Design review of the part built by this model. Coordinates are the model's own, in mm. Face numbers are marked on the shaded views. A direction names the side the tool comes from. Round coordinates to 2 decimals unless told otherwise and drop trailing zeros. Write each loop counter-clockwise with the first axis right and the second up, starting at its lowest first coordinate (ties: lowest second). Pieces come first, ordered by that corner, then holes. Notation, with made-up numbers: (15, -40) -> (34, -40) arc R29 cw to (34, -13) -> close; hole circle Ø10 at (-13, 26.5). An arc over 180 degrees is marked (long way). One line per question, with ' | ' between items. Start each with the question number.
1) Consider section C-C (x = 0). Give the boundary of the cut face in (y, z), then the cut area to 3 significant figures.
2) For the marked faces 1 and 2, list the 3-axis set-ups (+Z, -Z, +X, -X, +Y, -Y) from which the entire face can be reached by the end or side of a thin tool; tool diameter is ignored.
3) For probe 1 along X at (y, z) = (18, 0.25); probe 2 along Y at (x, z) = (9.75, -0.75); probe 3 along Z at (x, y) = (-8, 18), list the stretches that pass through material, from the lowest coordinate up.
4) Consider section B-B (x = -8). Give the boundary of the cut face in (y, z).
5) Consider section D-D (y = 26). Give the boundary of the cut face in (x, z), then the cut area to 3 significant figures.
6) Consider section A-A (z = 0). Give the boundary of the cut face in (x, y), then the cut area to 3 significant figures.
7) Insertion check: pin 1 Ø12 at (x, z) = (-4, 7.5) entering from -Y; pin 2 Ø3 at (x, y) = (11.5, 25.5) entering from -Z; pin 3 Ø2 at (x, z) = (12, -0.5) entering from -Y; pin 4 Ø9 at (x, z) = (-2.5, -1.5) entering from -Y. Each pin has a flat end and moves straight along its axis. Give the tip position at first contact, or say it passes through.
```python
from build123d import *

# Parameters (mm, degrees)
F0_R     = 15
F0_R_2   = 1.25
F0_R_3   = 5.5
F1_DEPTH = 45
F2_DEPTH = 2
F3_R     = 1.6
F4_DEPTH = 9


with BuildPart() as f1:
    # F0 (on Front) → F1 (new body)
    with BuildSketch(Plane.XZ):
        Circle(F0_R)
        with Locations((-8, 0)):
            Circle(F0_R_2, mode=Mode.SUBTRACT)
        Circle(F0_R_3, mode=Mode.SUBTRACT)
        with Locations((8, 0)):
            Circle(F0_R_2, mode=Mode.SUBTRACT)
        Circle(F0_R_3)
    extrude(amount=-F1_DEPTH)

    # F0 (on Front) → F2 (join)
    with BuildSketch(Plane.XZ):
        Circle(F0_R_3)
    extrude(amount=F2_DEPTH)

    # F3 (on face) → F4 (join)
    with BuildSketch(Plane.XZ.offset(2)):
        Circle(F3_R)
    extrude(amount=F4_DEPTH)


solid = f1.part
```
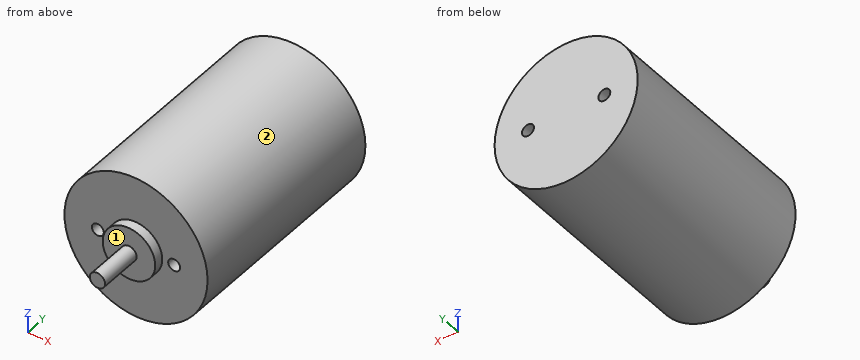
From the geometry:
1) outline: (-11, -1.6) -> (-2, -1.6) -> (-2, -5.5) -> (0, -5.5) -> (0, -15) -> (45, -15) -> (45, 15) -> (0, 15) -> (0, 5.5) -> (-2, 5.5) -> (-2, 1.6) -> (-11, 1.6) -> close | area: 1,400 mm2
2) face 1: -Y | face 2: +Y, -Y
3) probe 1: x = -15 to -9.22, -6.78 to 6.78, 9.22 to 15 | probe 2: y = 0 to 45 | probe 3: z = -12.69 to -1.25, 1.25 to 12.69
4) outline: (0, -12.69) -> (45, -12.69) -> (45, -1.25) -> (0, -1.25) -> close; (0, 1.25) -> (45, 1.25) -> (45, 12.69) -> (0, 12.69) -> close
5) outline: circle Ø30 at (0, 0); hole circle Ø2.5 at (-8, 0); hole circle Ø2.5 at (8, 0) | area: 697 mm2
6) outline: (-15, 0) -> (-9.25, 0) -> (-9.25, 45) -> (-15, 45) -> close; (-6.75, 0) -> (-5.5, 0) -> (-5.5, -2) -> (-1.6, -2) -> (-1.6, -11) -> (1.6, -11) -> (1.6, -2) -> (5.5, -2) -> (5.5, 0) -> (6.75, 0) -> (6.75, 45) -> (-6.75, 45) -> close; (9.25, 0) -> (15, 0) -> (15, 45) -> (9.25, 45) -> close | area: 1,180 mm2
7) pin 1: stops at y = -2 | pin 2: stops at z = -11.18 | pin 3: stops at y = 0 | pin 4: stops at y = -11
